The model under review builds one solid part; all positions refer to its coordinate system, in mm. A direction names the side the tool comes from. Round coordinates to 2 decimals unless told otherwise and drop trailing zeros. Write each loop counter-clockwise with the first axis right and the second up, starting at its lowest first coordinate (ties: lowest second). Pieces come first, ordered by that corner, then holes. Notation, with made-up numbers: M 78.25,-24 L 126.25,-24 A34 cw 126.25,12 Z; hole C 34,64 d8. An arc over 180 degrees is marked long. One line per item, written item: value. Start each with the question number.
1) Mouldability with a two-part tool opening along X and no side actions: class faces 3 (the face through (-1.71, 0.72, 3.04)), 4 (the face through (4, 0, 4.1)) as +X half, -X half, draft (parallel to the pull), parting line (faces both ways), or undercut.
2) For P1, Ø2, axis at x = 2, z = 2, coming from the -Y side; P2, Ø1.5, axis at x = -7.5, y = -5, coming from the +Z side; P3, Ø1.5, axis at x = -1.5, z = 1.5, coming from the -Y side, all flat-tipped, find the tip position at first contact; note any pin that passes through.
3) Tool access review of faces 1 (the face through (0, 0, 0)), 2 (the face through (0, 0, 2)): name each direction out of +Z, -Z, +X, -X, +Y, -Y from which nothing blocks a thin tool from reaching the whole face with its end or side.
4) Take a section at D-D, the plane z = 0.45. Write out the cut boundary in (x, y).
5) Take a section at B-B, the plane z = 2.5. Write out the cut boundary in (x, y).
6) Wall thickness on probe 1 along Z at (x, y) = (-6, -3.5); probe 2 along X at (y, z) = (0.25, 3.15); probe 3 along X at (y, z) = (2, 2.1): over which ranges is each line inside the solid? List them lowest first.
from build123d import *

# Parameters (mm, degrees)
F0_R     = 10
F1_DEPTH = 2
F2_R     = 1.99999
F3_R     = 2.4
F4_DEPTH = 2.1


# Not quite as in the source:
# - a fillet or chamfer is up to 0.001 mm smaller than in the source, because OpenCascade refuses the exact size


with BuildPart() as f1:
    # F0 (on Top) → F1 (new body)
    with BuildSketch(Plane.XY):
        Circle(F0_R)
    extrude(amount=F1_DEPTH)

    # F2 (radius 2 in the source; OpenCascade refuses exactly that, so slightly less here)
    f2_edges = [f1.edges().sort_by_distance(p)[0] for p in [
        (-10, 0, 2),
    ]]
    fillet(f2_edges, radius=F2_R)

    # F3 (on face) → F4 (join)
    with BuildSketch(Plane.XY.offset(2)):
        with Locations((-4, 0)):
            Circle(F3_R)
        with Locations((4, 0)):
            Circle(F3_R)
    extrude(amount=F4_DEPTH)


solid = f1.part
Checked values:
1. face 3: undercut
1. face 4: draft
2. P1: stops at y = -9.55
2. P2: stops at z = 1.98
2. P3: stops at y = -9.76
3. face 1: -Z, +X, -X, +Y, -Y
3. face 2: +Z
4. outline: C 0,0 d19.9
5. outline: C -4,0 d4.8; C 4,0 d4.8
6. probe 1: z = 0 to 2
6. probe 2: x = -6.39 to -1.61, 1.61 to 6.39
6. probe 3: x = -5.33 to -2.67, 2.67 to 5.33
